Answer from the drawing. Dimensions are ordinates in mm from the lowest x, y and z of the part. Give positions to 0.01 mm unless a question says otherwise; leave off trailing zeros. Loops run counter-clockwise (first coordinate to the right, second up) from the corner with the lowest first, then second, coordinate; pieces in that order, holes last. Notation, with made-up numbers: (13.25, 65) - (33.25, 65) arc R21 ccw to (33.25, 97) - close; hole circle Ø7 at (-6.75, 70.5). An arc over 180 degrees is marked (long way). Put each result on its own line as item: value. Start each with the question number.
1. Given pin 1 Ø1.5 at (x, y) = (61.5, 7.5) entering from -Z, flat-ended and moving along its own axis, determine where the tip first touches the part or whether it passes through.
2. Consider L1, parallel to X at y = 4.5, z = 59.5; L2, parallel to X at y = 3.5, z = 59 (1 decimal); L3, parallel to Z at x = 20.5, y = 9. Determine where each line is inside the solid, lowest interval first. Write a range as from..to.
3. A cutting plane is placed at A-A, the plane z = 63. Determine the outline of the cut face in (x, y) (1 decimal), plus the area to 3 significant figures.
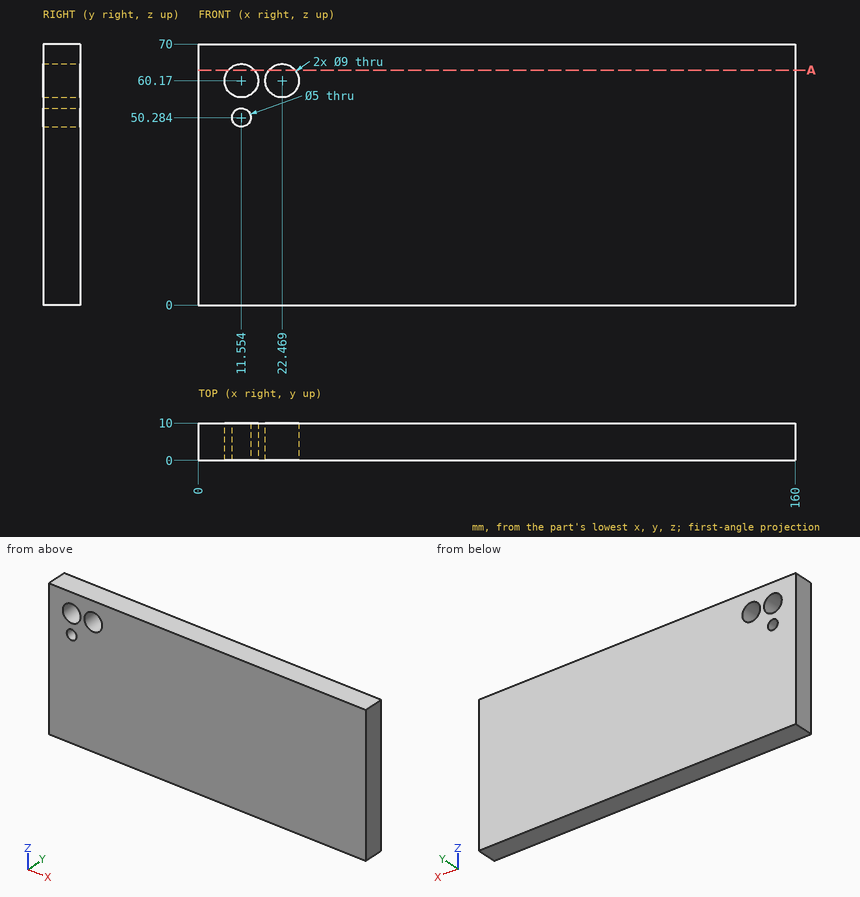
Return value:
1. pin 1: stops at z = 0
2. L1: x = 0..7.1, 16..18.02, 26.92..160
2. L2: x = 0..7.2, 15.9..18.1, 26.8..160
2. L3: z = 0..56.12, 64.22..70
3. outline: (0, 0) - (8.1, 0) - (8.1, 10) - (0, 10) - close; (15.1, 0) - (19, 0) - (19, 10) - (15.1, 10) - close; (26, 0) - (160, 0) - (160, 10) - (26, 10) - close
3. area: 1,460 mm2
